CAD build for the part. Positions are in the model's coordinates, mm. Face numbers are marked on the shaded views. A direction names the side the tool comes from. Give positions to 0.01 mm unless a question says otherwise; leave off trailing zeros. Write each loop counter-clockwise with the first axis right and the second up, starting at its lowest first coordinate (ties: lowest second). Pieces come first, ordered by that corner, then holes. Notation, with made-up numbers: (64.25, 67) - (68.25, 67) arc R32 cw to (68.25, 95) - close; hole circle Ø4 at (-19, 30). An arc over 180 degrees is marked (long way). Answer as a JSON object with one key per item and string values.
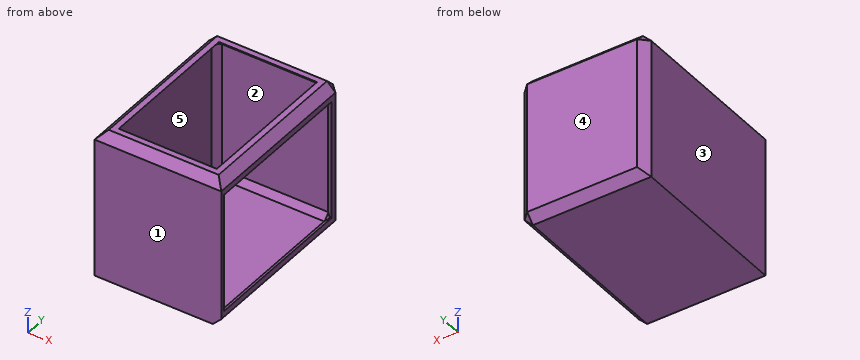
from build123d import *

# Parameters (mm, degrees)
F1_W     = 76.656278
F1_H     = 89.442563
F2_DEPTH = 105.492987
F4_SIZE  = 5.08
F5_T     = -2.54


with BuildPart() as f2:
    # F1 (on face) → F2 (new body)
    with BuildSketch(Plane.XZ):
        with Locations((-9.342497, 12.035428)):
            Rectangle(F1_W, F1_H)
    extrude(amount=F2_DEPTH)

    # F4
    f4_edges = [f2.edges().sort_by_distance(p)[0] for p in [
        (-9.342497, 0, 56.756709),
        (28.985642, -52.746493, 56.756709),
        (-47.670636, -52.746493, 56.756709),
        (-9.342497, -105.492987, 56.756709),
        (-9.342497, 0, -32.685854),
        (28.985642, 0, 12.035428),
        (-47.670636, 0, 12.035428),
        (28.985642, -52.746493, -32.685854),
    ]]
    chamfer(f4_edges, length=F4_SIZE)

    # F5
    f5_openings = [f2.faces().sort_by_distance(p)[0] for p in [
        (28.985642, -55.286493, 12.035428),
        (-9.342497, -52.746493, 56.756709),
    ]]
    offset(amount=F5_T, openings=f5_openings)


solid = f2.part
Item 1: Cut at B-B (x = 18.5). Give the cut face in (y, z), and give its area (3 significant figures).
Entries:
{"outline": "(-105.49, -32.69) - (-5.08, -32.69) - (0, -27.61) - (0, 51.68) - (-5.08, 56.76) - (-8.67, 56.76) - (-2.54, 50.62) - (-2.54, -26.55) - (-6.13, -30.15) - (-102.95, -30.15) - (-102.95, 50.62) - (-96.82, 56.76) - (-100.41, 56.76) - (-105.49, 51.68) - close", "area": "715 mm2"}
Item 2: Cut at A-A (y = -76.5). Give the cut face in (x, z), and give its area (3 significant figures).
Entries:
{"outline": "(-47.67, -32.69) - (23.91, -32.69) - (28.99, -27.61) - (28.99, -24.01) - (22.85, -30.15) - (-45.13, -30.15) - (-45.13, 50.62) - (-39, 56.76) - (-42.59, 56.76) - (-47.67, 51.68) - close; (20.31, 56.76) - (28.99, 48.08) - (28.99, 51.68) - (23.91, 56.76) - close", "area": "452 mm2"}
Item 3: Cut at C-C (z = 37). Give the cut face in (x, y).
Entries:
{"outline": "(-47.67, -105.49) - (28.99, -105.49) - (28.99, -102.95) - (-45.13, -102.95) - (-45.13, -6.13) - (-41.54, -2.54) - (22.85, -2.54) - (28.99, -8.67) - (28.99, -5.08) - (23.91, 0) - (-42.59, 0) - (-47.67, -5.08) - close"}
Item 4: Mould opens along Y. For the marked faces 3, 4 and 5 say: +Y half, -Y half, draft (parallel to the pull), parting line (faces both ways), or undercut.
Entries:
{"face 3": "draft", "face 4": "+Y half", "face 5": "undercut"}
Item 5: Probe line 1 (Y direction, x = -17, z = 32.5); line 2 (X direction, y = -73, z = -15); line 3 (Z direction, x = -8.5, y = -52). List the from-to ranges inside material, lowest first. Write a range as from..to.
Entries:
{"line 1": "-105.49..-102.95, -2.54..0", "line 2": "-47.67..-45.13", "line 3": "-32.69..-30.15"}
Item 6: Which spindle directions (+Z, -Z, +X, -X, +Y, -Y) get a long thin tool onto all of the face, cutting with end or side? Do the marked faces 1 and 2. Say none if no direction does.
Entries:
{"face 1": "+Z, -Z, +X, -X, -Y", "face 2": "none"}
Item 7: Flat gauge pins, fed straight in: P1, Ø6, axis at y = -69.5, z = 24, coming from the +X side; P2, Ø3, axis at x = 0, y = -51.5, coming from the +Z side. Where does each tip first touch, or does it go through?
Entries:
{"P1": "x = -45.13", "P2": "z = -30.15"}
